For this review, take the finished solid that the model builds, in its own axes (mm). A direction names the side the tool comes from. Coordinates: 2 decimals unless noted, no trailing zeros. Order: outer loops, then holes, each group sorted by start corner. A loop starts at its lowest first (then second) coordinate and runs counter-clockwise, first axis right, second up. Notation, with made-up numbers: (73.5, 33) -> (77.5, 33) arc R30 ccw to (77.5, 62) -> close; hole circle Ø11 at (77.25, -35.75). An arc over 180 degrees is marked (long way). Return JSON: item names as keys, results as strings. Group by question number.
Item 1: Draft analysis for pull direction Y (two halves, no side actions). For faces 1 (the flat face through (5, 6, 5.7)), 2 (the cylindrical face through (0.752, 59.287, 4.437)), state which applies: +Y half, -Y half, draft (parallel to the pull), parting line (faces both ways), or undercut.
Item 2: Take a section at A-A (y = 13). Write out the cut boundary in (x, z), then the cut area to 3 significant figures.
Item 3: Take a section at C-C (z = 8). Count the separate pieces of the cut face and the enclosed holes in it, then the cut area to 3 significant figures.
Item 4: Take a section at D-D (x = 27). Write out the cut boundary in (y, z), then the cut area to 3 significant figures.
Item 5: For line 1 along Y through (x, z) = (-2, 5.25); line 2 along Y through (x, z) = (70, 4.55); line 3 along Y through (x, z) = (47, 4.5), list the stretches that pass through material, from the lowest coordinate up.
Item 6: Machinability: for faces 3 (the cylindrical face through (-0.57, 41.4, 4.44)), 4 (the flat face through (63, 55, 5.7)), 5 (the flat face through (20, 30, 1)), which of the approach directions +Z, -Z, +X, -X, +Y, -Y give a long, thin tool a straight path to every point of the face, cutting with its end or side? Answer none if there is none.
Item 7: Take a section at B-B (x = 83.5). Write out the cut boundary in (y, z).
Item 8: Insertion check: pin 1 (2 mm diameter, centred on x = 60.5, y = 51.5, fed in from +Z); pin 2 (3 mm diameter, centred on x = 6.5, y = 55.5, fed in from +Z); pin 3 (1.6 mm diameter, centred on y = 27.5, z = 0.5, fed in from -X). Each pin has a flat end and moves straight along its axis. Give the tip position at first contact, or say it passes through.
```python
from build123d import *

# Parameters (mm, degrees)
SKETCH_R        = 1.8
PAD_DEPTH       = 9
POCKET_DEPTH    = 7
SKETCH002_R     = 3.1
SKETCH002_W     = 2
SKETCH002_H     = 52
PAD001_DEPTH    = 2.7
SKETCH003_R     = 1
PAD002_DEPTH    = 1
POCKET001_DEPTH = 2
POCKET002_DEPTH = 2
SKETCH006_R     = 3.5
POCKET003_DEPTH = 5
POCKET004_DEPTH = 3
SKETCH009_W     = 5
SKETCH009_H     = 30
POCKET005_DEPTH = 5


with BuildPart() as part:
    # Sketch → Pad (new body)
    with BuildSketch(Plane.XY):
        with BuildLine():
            Line((89.002639, 2.5), (89.002639, 57.5))
            ThreePointArc((89.002639, 57.5), (88.270406, 59.267767), (86.502639, 60))
            Line((77, 60), (86.502639, 60))
            ThreePointArc((75, 62), (75.585786, 60.585786), (77, 60))
            ThreePointArc((75, 62), (70, 67), (65, 62))
            ThreePointArc((63, 60), (64.414214, 60.585786), (65, 62))
            Line((2.5, 60), (63, 60))
            ThreePointArc((2.5, 60), (0.732233, 59.267767), (0, 57.500001))
            Line((0, 57.500001), (0, 54))
            ThreePointArc((-2, 52), (-0.585786, 52.585786), (0, 54))
            ThreePointArc((-2, 52), (-7, 47), (-2, 42))
            ThreePointArc((0, 40), (-0.585786, 41.414214), (-2, 42))
            Line((0, 40), (0, 20))
            ThreePointArc((-2, 18), (-0.585786, 18.585786), (0, 20))
            ThreePointArc((-2, 18), (-7, 13), (-2, 8))
            ThreePointArc((0, 6), (-0.585786, 7.414214), (-2, 8))
            Line((0, 6), (0, 2.499999))
            ThreePointArc((0, 2.499999), (0.732233, 0.732233), (2.5, 0))
            Line((2.5, 0), (63, 0))
            ThreePointArc((65, -2), (64.414214, -0.585786), (63, 0))
            ThreePointArc((65, -2), (70, -7), (75, -2))
            ThreePointArc((77, 0), (75.585786, -0.585786), (75, -2))
            Line((77, 0), (86.502639, 0))
            ThreePointArc((86.502639, 0), (88.270406, 0.732233), (89.002639, 2.5))
        make_face()
        with Locations((70, 62)):
            Circle(SKETCH_R, mode=Mode.SUBTRACT)
        with Locations((-2, 47)):
            Circle(SKETCH_R, mode=Mode.SUBTRACT)
        with Locations((-2, 13)):
            Circle(SKETCH_R, mode=Mode.SUBTRACT)
        with Locations((70, -2)):
            Circle(SKETCH_R, mode=Mode.SUBTRACT)
    extrude(amount=PAD_DEPTH)

    # Sketch001 → Pocket (cut)
    with BuildSketch(Plane.XY.offset(9)):
        with BuildLine():
            Line((87.5, 3.2), (87.5, 56.8))
            ThreePointArc((87.5, 56.8), (87.002082, 58.002081), (85.8, 58.5))
            Line((3.199992, 58.5), (85.8, 58.5))
            ThreePointArc((3.199992, 58.5), (1.997916, 58.002079), (1.5, 56.8))
            Line((1.5, 56.8), (1.5, 3.2))
            ThreePointArc((1.5, 3.2), (1.997916, 1.997921), (3.199992, 1.5))
            Line((3.199992, 1.5), (85.8, 1.5))
            ThreePointArc((85.8, 1.5), (87.002082, 1.997918), (87.5, 3.2))
        make_face()
    extrude(amount=-POCKET_DEPTH, mode=Mode.SUBTRACT)

    # Sketch002 → Pad001 (new body)
    with BuildSketch(Plane.XY.offset(2)):
        with Locations((5.5, 5.5)):
            Circle(SKETCH002_R)
        with Locations((5.5, 54.5)):
            Circle(SKETCH002_R)
        with Locations((63.5, 54.5)):
            Circle(SKETCH002_R)
        with Locations((63.5, 5.5)):
            Circle(SKETCH002_R)
        with Locations((86, 30)):
            Rectangle(SKETCH002_W, SKETCH002_H)
    extrude(amount=PAD001_DEPTH)

    # Sketch003 → Pad002 (new body)
    with BuildSketch(Plane.XY.offset(4.7)):
        with Locations((5.5, 54.5)):
            Circle(SKETCH003_R)
        with Locations((63.5, 54.5)):
            Circle(SKETCH003_R)
        with Locations((63.5, 5.5)):
            Circle(SKETCH003_R)
        with Locations((5.5, 5.5)):
            Circle(SKETCH003_R)
    extrude(amount=PAD002_DEPTH)

    # Sketch004 → Pocket001 (cut)
    with BuildSketch(Plane(origin=(0, 0, 0), x_dir=(0, -1, 0), z_dir=(-1, 0, 0))):
        Polygon((-37.5, 9), (-22.5, 9), (-22.5, 0), (-30, 0), (-37.5, 0), align=None)
    extrude(amount=-POCKET001_DEPTH, mode=Mode.SUBTRACT)

    # Sketch005 → Pocket002 (cut)
    with BuildSketch(Plane.YZ.offset(89.002639)):
        Polygon((3, 9), (57, 9), (57, 6), (30, 6), (3, 6), align=None)
    extrude(amount=-POCKET002_DEPTH, mode=Mode.SUBTRACT)

    # Sketch006 → Pocket003 (cut)
    with BuildSketch(Plane.XZ):
        with Locations((55.5, 9)):
            Circle(SKETCH006_R)
        Polygon((42, 5.5), (42, 13.5), (26, 13.5), (26, 5.5), (34, 5.5), align=None)
        Polygon((17.1, 5.5), (17.1, 9), (8.1, 9), (8.1, 5.5), (12.6, 5.5), align=None)
    extrude(amount=-POCKET003_DEPTH, mode=Mode.SUBTRACT)

    # Sketch008 → Pocket004 (cut)
    with BuildSketch(Plane(origin=(0, 0, 0), x_dir=(1, 0, 0), z_dir=(0, 0, -1))):
        Polygon((-5, -14.732051), (-5, -11.267949), (-2, -9.535898), (1, -11.267949), (1, -14.732051), (-2, -16.464102), align=None)
        Polygon((-5, -48.732051), (-5, -45.267949), (-2, -43.535898), (1, -45.267949), (1, -48.732051), (-2, -50.464102), align=None)
        Polygon((67, 0.267949), (67, 3.732051), (70, 5.464102), (73, 3.732051), (73, 0.267949), (70, -1.464102), align=None)
        Polygon((67, -63.732051), (67, -60.267949), (70, -58.535898), (73, -60.267949), (73, -63.732051), (70, -65.464102), align=None)
    extrude(amount=-POCKET004_DEPTH, mode=Mode.SUBTRACT)

    # Sketch009 → Pocket005 (cut)
    with BuildSketch(Plane.XY.offset(2)):
        Polygon((10, 15), (15, 15), (15, 45), (10, 45), (10, 30), align=None)
        with Locations((22.5, 30)):
            Rectangle(SKETCH009_W, SKETCH009_H)
        with Locations((32.5, 30)):
            Rectangle(SKETCH009_W, SKETCH009_H)
        with Locations((42.5, 30)):
            Rectangle(SKETCH009_W, SKETCH009_H)
        with Locations((52.5, 30)):
            Rectangle(SKETCH009_W, SKETCH009_H)
    extrude(amount=-POCKET005_DEPTH, mode=Mode.SUBTRACT)


solid = part.part
```
Findings below:
{
 "1": {"face 1": "undercut", "face 2": "+Y half"},
 "2": {"outline": "(-7, 0) -> (-5, 0) -> (-5, 3) -> (-3.8, 3) -> (-3.8, 9) -> (-7, 9) -> close; (-0.2, 3) -> (1, 3) -> (1, 0) -> (89, 0) -> (89, 6) -> (87.5, 6) -> (87.5, 2) -> (87, 2) -> (87, 4.7) -> (85, 4.7) -> (85, 2) -> (1.5, 2) -> (1.5, 9) -> (-0.2, 9) -> close", "area": "223 mm2"},
 "3": {"separate pieces": "5", "enclosed holes": "4", "area": "487 mm2"},
 "4": {"outline": "(0, 0) -> (60, 0) -> (60, 9) -> (58.5, 9) -> (58.5, 2) -> (1.5, 2) -> (1.5, 5.5) -> (0, 5.5) -> close", "area": "136 mm2"},
 "5": {"line 1": "y = 8 to 11.2, 14.8 to 18, 42 to 45.2, 48.8 to 52", "line 2": "y = -7 to -3.8, -0.2 to 1.5, 58.5 to 60.2, 63.8 to 67", "line 3": "y = 0 to 1.5, 58.5 to 60"},
 "6": {"face 3": "+Z, -Z, -X", "face 4": "+Z", "face 5": "+Z, -Z"},
 "7": {"outline": "(0, 0) -> (60, 0) -> (60, 9) -> (58.5, 9) -> (58.5, 2) -> (1.5, 2) -> (1.5, 9) -> (0, 9) -> close"},
 "8": {"pin 1": "stops at z = 2", "pin 2": "stops at z = 5.7", "pin 3": "stops at x = 2"}
}
